Can you work these out from the model? Positions are in its coordinate system, mm. A direction names the side the tool comes from. Coordinates: 2 decimals unless noted, no trailing zeros. Order: outer loops, then holes, each group sorted by start corner. A loop starts at its lowest first (then second) coordinate and runs counter-clockwise, first axis right, second up. Notation, with made-up numbers: (69.25, 5.25) -> (81.25, 5.25) arc R23 cw to (81.25, 25.25) -> close; hole circle Ø7 at (43.25, -17.75). An arc over 180 degrees is marked (long way). Answer as a JSON object with one key per item and string values. Group by question number.
(1) I want a section at D-D, the plane y = 3.75. List the corners of the cut face in (x, z) for me, plus the area to 3 significant figures.
(2) I want a section at C-C, the plane y = 1.25. List the corners of the cut face in (x, z) for me.
(3) For pin 1 (7 mm diameter, centred on x = 0, z = 0, fed in from -Y); pin 2 (1 mm diameter, centred on x = -5.5, y = 3, fed in from -Z); pin 3 (1 mm diameter, centred on y = 6, z = 7, fed in from +X), each with a flat end and sliding along its axis, tell me the tip position at first contact or that it passes through.
(4) I need wall thicknesses on line 1 (Z direction, x = 0, y = 0.75); line 2 (Z direction, x = 1, y = 4); line 3 (Y direction, x = -8, z = 1.25). Which ranges of each line are inside material? Lowest first, please.
(5) If we mould it in two halves opening along X, with no side actions, what happens to faces 3 (the flat face through (0, 7, -2)), 4 (the cylindrical face through (2.01, 5.26, -9.03)), 5 (the cylindrical face through (-6, 1, 0))? For each: pulls with the +X half, pulls with the -X half, needs draft (parallel to the pull), parting line crosses it, or undercut.
(6) I want a section at B-B, the plane x = 0. List the corners of the cut face in (y, z) for me.
(7) I want a section at A-A, the plane z = 0. List the corners of the cut face in (x, y) for me, plus the area to 3 significant figures.
(8) Which directions (+Z, -Z, +X, -X, +Y, -Y) give clear straight access to the entire face, cutting with the end or side of a thin tool? Please do faces 1 (the cylindrical face through (2.01, 0.76, -9.03)), 2 (the flat face through (6, 0, -2)).
from build123d import *

# Parameters (mm, degrees)
SKETCH4_R                 = 6
CUT_EXTRUDE1_DEPTH        = 3
M4X0_7_TAPPED_HOLE1_D     = 3.3
M4X0_7_TAPPED_HOLE1_DEPTH = 4
M4X0_7_TAPPED_HOLE1_TIP   = 0.991420021


with BuildPart() as part:
    # Sketch1 → Revolve1 (revolve)
    with BuildSketch(Plane.XY):
        with BuildLine():
            Line((0, 0), (-9.25, 0))
            Line((-9.25, 0), (-9.25, 1.5))
            ThreePointArc((-9.25, 1.5), (-7.75, 3), (-9.25, 4.5))
            Line((-9.25, 4.5), (-9.25, 6))
            Line((-9.25, 6), (-9.75, 6))
            Line((-9.75, 6), (-9.75, 7))
            Line((-9.75, 7), (0, 7))
            Line((0, 7), (0, 0))
        make_face()
    revolve(axis=Axis((0, 0, 0), (0, 1, 0)))

    # Sketch4 → Cut-Extrude1 (cut)
    with BuildSketch(Plane.XZ):
        Circle(SKETCH4_R)
    extrude(amount=-CUT_EXTRUDE1_DEPTH, mode=Mode.SUBTRACT)

    # M4x0.7 Tapped Hole1
    with Locations(Plane(origin=(0, 7, 0), x_dir=(1, 0, 0), z_dir=(0, 1, 0))):
        with Locations((0, 0)):
            Hole(M4X0_7_TAPPED_HOLE1_D / 2, depth=M4X0_7_TAPPED_HOLE1_DEPTH)
            with Locations((0, 0, -(M4X0_7_TAPPED_HOLE1_DEPTH + M4X0_7_TAPPED_HOLE1_TIP / 2))):  # 118° drill point
                Cone(0, M4X0_7_TAPPED_HOLE1_D / 2, M4X0_7_TAPPED_HOLE1_TIP, mode=Mode.SUBTRACT)


solid = part.part
Computed values:
{
 "1": {"outline": "circle Ø15.9 at (0, 0); hole circle Ø3.3 at (0, 0)", "area": "190 mm2"},
 "2": {"outline": "circle Ø18.5 at (0, 0); hole circle Ø12 at (0, 0)"},
 "3": {"pin 1": "stops at y = 3", "pin 2": "stops at z = -5.92", "pin 3": "stops at x = 7.27"},
 "4": {"line 1": "z = -9.25 to -6, 6 to 9.25", "line 2": "z = -8.07 to -1.31, 1.31 to 8.07", "line 3": "y = 0 to 2.04, 3.96 to 7"},
 "5": {"face 3": "needs draft", "face 4": "parting line crosses it", "face 5": "undercut"},
 "6": {"outline": "(0, -9.25) -> (1.5, -9.25) arc R1.5 cw to (4.5, -9.25) -> (6, -9.25) -> (6, -9.75) -> (7, -9.75) -> (7, -1.65) -> (3, -1.65) -> (3, -6) -> (0, -6) -> close; (0, 6) -> (3, 6) -> (3, 1.65) -> (7, 1.65) -> (7, 9.75) -> (6, 9.75) -> (6, 9.25) -> (4.5, 9.25) arc R1.5 cw to (1.5, 9.25) -> (0, 9.25) -> close"},
 "7": {"outline": "(-9.75, 6) -> (-9.25, 6) -> (-9.25, 4.5) arc R1.5 cw to (-9.25, 1.5) -> (-9.25, 0) -> (-6, 0) -> (-6, 3) -> (-1.65, 3) -> (-1.65, 7) -> (-9.75, 7) -> close; (1.65, 3) -> (6, 3) -> (6, 0) -> (9.25, 0) -> (9.25, 1.5) arc R1.5 cw to (9.25, 4.5) -> (9.25, 6) -> (9.75, 6) -> (9.75, 7) -> (1.65, 7) -> close", "area": "74.2 mm2"},
 "8": {"face 1": "-Y", "face 2": "+Z, -Z, +X, -X, -Y"}
}
